Work out the finished part from the listing and answer in its coordinate system (mm). A direction names the side the tool comes from. Coordinates: 2 decimals unless noted, no trailing zeros. Order: outer loops, then holes, each group sorted by start corner. A loop starts at its lowest first (then second) coordinate and runs counter-clockwise, first axis right, second up. Notation, with made-up numbers: (57.5, -16.5) - (71.5, -16.5) arc R18 ccw to (71.5, -2.5) - close; hole circle Ø4 at (82, 62.5). An arc over 180 degrees is marked (long way). Answer as a JSON object with one key per item and string values. Group by question number.
1) A tool of negligible diameter and unlimited length cuts with its end or side. For faces 1 (the face through (1, -1, 3)), 2 (the face through (-1.352, 4, 2)), 3 (the face through (-0.38, 40.5, 2.48)), 4 (the face through (1.952, 3, 2)), 5 (the face through (-0.217, -0.976, -0.507)), from which of +Z, -Z, +X, -X, +Y, -Y can it reach the whole face along a straight path? Write none if from no direction.
2) Section B-B (y = 0) is taken. Give the vertices of the cut face in (x, z), plus the area to 3 significant figures.
3) Section C-C (z = 1.6) is taken. Give the vertices of the cut face in (x, y).
4) Each of these flat-tipped pins is pushed along its axis until it touches: P1, Ø2.5, axis at y = 4, z = 1.5, coming from the +X side; P2, Ø1.5, axis at x = 1.5, y = 20, coming from the -Z side; P3, Ø1, axis at x = -2, z = 1.5, coming from the +Y side. Where does it stop, or does it pass through?
5) Section D-D (y = 62) is taken. Give the vertices of the cut face in (x, z).
6) Find the intervals of material crossed by line 1 along X through (y, z) = (38, 1.5); line 2 along Z through (x, y) = (0.1, 69.5); line 3 along Z through (x, y) = (0.4, 51), in increasing order.
from build123d import *

# Parameters (mm, degrees)
SKETCH1_R                = 2.49
BOSS_EXTRUDE1_DEPTH      = 3
BOSS_EXTRUDE2_DEPTH      = 1
BOSS_EXTRUDE2_DEPTH_BACK = 4
SKETCH2_R                = 1
SKETCH3_W                = 3.303783413
SKETCH3_H                = 2.177091536
BOSS_EXTRUDE3_DEPTH      = 5
SKETCH4_R                = 1
BOSS_EXTRUDE4_DEPTH      = 72


with BuildPart() as part:
    # Sketch1 → Boss-Extrude1 (new body)
    with BuildSketch(Plane.XY):
        Circle(SKETCH1_R)
    extrude(amount=BOSS_EXTRUDE1_DEPTH)

    # Sketch2 → Boss-Extrude2 (add, two sides: drawn at the far end of the back side and taken through both)
    with BuildSketch(Plane.XY.offset(3).offset(-BOSS_EXTRUDE2_DEPTH_BACK)):
        Circle(SKETCH2_R)
    extrude(amount=BOSS_EXTRUDE2_DEPTH + BOSS_EXTRUDE2_DEPTH_BACK)

    # Sketch3 → Boss-Extrude3 (add)
    with BuildSketch(Plane(origin=(0, 0, 0), x_dir=(1, 0, 0), z_dir=(0, 1, 0))):
        with Locations((0.300293678, -1.5)):
            Rectangle(SKETCH3_W, SKETCH3_H)
    extrude(amount=BOSS_EXTRUDE3_DEPTH)

    # Sketch4 → Boss-Extrude4 (add)
    with BuildSketch(Plane(origin=(0, 5, 0), x_dir=(1, 0, 0), z_dir=(0, 1, 0))):
        with Locations(Location((0, -1.555640041, 0), (0, 0, 270))):
            Circle(SKETCH4_R)
    extrude(amount=BOSS_EXTRUDE4_DEPTH)


solid = part.part
Report:
{
 "1": {"face 1": "+Z", "face 2": "+Z, -Z, -X, +Y", "face 3": "+Y", "face 4": "+Z, -Z, +X, +Y", "face 5": "-Z"},
 "2": {"outline": "(-2.49, 0) - (-1, 0) - (-1, -1) - (1, -1) - (1, 0) - (2.49, 0) - (2.49, 3) - (1, 3) - (1, 4) - (-1, 4) - (-1, 3) - (-2.49, 3) - close", "area": "18.9 mm²"},
 "3": {"outline": "(-1.35, 2.09) arc R2.49 ccw (long way) to (1.95, 1.55) - (1.95, 5) - (1, 5) - (1, 77) - (-1, 77) - (-1, 5) - (-1.35, 5) - close"},
 "4": {"P1": "stops at x = 1.95", "P2": "stops at z = 0.89", "P3": "stops at y = 1.99"},
 "5": {"outline": "circle Ø2 at (0, 1.56)"},
 "6": {"line 1": "x = -1 to 1", "line 2": "z = 0.56 to 2.55", "line 3": "z = 0.64 to 2.47"}
}
